For this review, take the finished solid that the model builds, in its own axes (mm). A direction names the side the tool comes from. Give positions to 0.01 mm unless a question says otherwise; leave off trailing zeros. Order: outer loops, then holes, each group sorted by start corner. A loop starts at its lowest first (then second) coordinate and runs counter-clockwise, first axis right, second up.
from build123d import *

# Parameters (mm, degrees)
SKETCH1_W           = 160
SKETCH1_H           = 110
SKETCH1_W_2         = 150
SKETCH1_H_2         = 100
BOSS_EXTRUDE1_DEPTH = 100
SKETCH2_R           = 5
CUT_EXTRUDE1_DEPTH  = 240
SKETCH3_R           = 5
CUT_EXTRUDE2_DEPTH  = 10


with BuildPart() as part:
    # Sketch1 → Boss-Extrude1 (new body)
    with BuildSketch(Plane.XY):
        with Locations((80, -55)):
            Rectangle(SKETCH1_W, SKETCH1_H)
        with Locations((80, -55)):
            Rectangle(SKETCH1_W_2, SKETCH1_H_2, mode=Mode.SUBTRACT)
    extrude(amount=BOSS_EXTRUDE1_DEPTH)

    # Sketch2 → Cut-Extrude1 (cut)
    with BuildSketch(Plane.XZ.offset(110)):
        with Locations(Location((40, 50, 0), (0, 0, 270))):
            Circle(SKETCH2_R)
    extrude(amount=-CUT_EXTRUDE1_DEPTH, mode=Mode.SUBTRACT)

    # Sketch3 → Cut-Extrude2 (cut)
    with BuildSketch(Plane(origin=(160, 0, 0), x_dir=(0, 0, -1), z_dir=(1, 0, 0))):
        with Locations(Location((-50, -60, 0), (0, 0, 90))):
            Circle(SKETCH3_R)
    extrude(amount=-CUT_EXTRUDE2_DEPTH, mode=Mode.SUBTRACT)


solid = part.part
1) Clearance check with a flat-ended pin moving along its axis: pin 1 (8 mm diameter, centred on x = 40, z = 50, fed in from +Y) (1 decimal). State where the tip first meets the part, or that it passes through.
Answer sheet:
pin 1: passes through
2) We need section D-D on x = 73. Give the boundary of the cut face in (y, z).
Answer sheet:
outline: (-110, 0) - (-105, 0) - (-105, 100) - (-110, 100) - close; (-5, 0) - (0, 0) - (0, 100) - (-5, 100) - close
3) We need section C-C on y = -69. Give the boundary of the cut face in (x, z).
Answer sheet:
outline: (0, 0) - (5, 0) - (5, 100) - (0, 100) - close; (155, 0) - (160, 0) - (160, 100) - (155, 100) - close
4) We need section B-B on x = 40. Give the boundary of the cut face in (y, z), then the cut area to 3 significant figures.
Answer sheet:
outline: (-110, 0) - (-105, 0) - (-105, 45) - (-110, 45) - close; (-110, 55) - (-105, 55) - (-105, 100) - (-110, 100) - close; (-5, 0) - (0, 0) - (0, 45) - (-5, 45) - close; (-5, 55) - (0, 55) - (0, 100) - (-5, 100) - close
area: 900 mm2
5) Tool access review of faces 4 (the face through (43, -3, 54)), 5 (the face through (157.535, -60.651, 54.957)), 6 (the face through (79, -105, 49)): name each direction out of +Z, -Z, +X, -X, +Y, -Y from which nothing blocks a thin tool from reaching the whole face with its end or side.
Answer sheet:
face 4: +Y, -Y
face 5: +X
face 6: +Z, -Z
6) To check wall thickness, follow line 1 (Y direction, x = 30, z = 11); line 2 (X direction, y = -106.2, z = 50); line 3 (X direction, y = -33, z = 54.5). State the ranges of each line that lie inside material, in increasing order.
Answer sheet:
line 1: y = -110 to -105, -5 to 0
line 2: x = 0 to 35, 45 to 160
line 3: x = 0 to 5, 155 to 160
7) Draft analysis for pull direction Y (two halves, no side actions). For faces 1 (the face through (79, 0, 49)), 2 (the face through (160, -56, 38)), 3 (the face through (5, -56, 49)), state which applies: +Y half, -Y half, draft (parallel to the pull), parting line (faces both ways), or undercut.
Answer sheet:
face 1: +Y half
face 2: draft
face 3: undercut
8) We need section A-A on z = 50. Give the boundary of the cut face in (x, y).
Answer sheet:
outline: (0, -110) - (35, -110) - (35, -105) - (5, -105) - (5, -5) - (35, -5) - (35, 0) - (0, 0) - close; (45, -110) - (160, -110) - (160, -65) - (155, -65) - (155, -105) - (45, -105) - close; (45, -5) - (155, -5) - (155, -55) - (160, -55) - (160, 0) - (45, 0) - close
